Check sheet for the modelled part. Datum: model origin and axes. Units: mm. A direction names the side the tool comes from. Coordinates: 2 decimals unless noted, no trailing zeros. Write each loop counter-clockwise with the first axis right and the second up, starting at its lowest first coordinate (ties: lowest second). Pieces come first, ordered by that corner, then holes. Notation, with made-up numbers: M 43,28 L 84,28 A9 cw 84,44 Z; hole C 42.5,80 d7. An arc over 180 degrees is marked long. Answer as CSV lines item,"result". Start each with the question number.
Q1. Sectioned sample at D-D, the plane x = -24. Count the separate pieces of the cut face and the enclosed holes in it, then the cut area to 3 significant figures.
Q2. Sectioned sample at A-A, the plane y = -24. Record the cut outline in (x, z) (3 decimals), then the cut area to 3 significant figures.
Q3. Depth check by flat-ended pin: pin 1 Ø2 at (x, y) = (-29, -7.5) entering from +Z; pin 2 Ø1 at (x, z) = (-21.5, -27) entering from -Y; pin 3 Ø1.5 at (x, y) = (9.5, -14.5) entering from -Z. Enter the tip coordinate at first touch or a pass-through.
Q4. Mould release check, pull along Z, two halves, no side actions. Record for faces 4 (the flat face through (0, -15, 31.5)), 5 (the flat face through (-29, -7, 53.501)), 6 (the flat face through (20, -15, 10)), 7 (the flat face through (0.2, -26.25, 33.6)): pulls with the +Z half, pulls with the -Z half, needs draft (parallel to the pull), parting line crosses it, or undercut.
Q5. Sectioned sample at C-C, the plane y = -15.5. Record the cut outline in (x, z) (3 decimals).
Q6. Access from +Z, -Z, +X, -X, +Y, -Y to the whole of each face (thin tool, end or side, straight path). Record for faces 1 (the flat face through (29, -7, 53.501)), 2 (the flat face through (-23, -22, -13.501)), 3 (the cylindrical face through (0.06, -28.59, -23.75)).
Q7. Thickness scan on line 1 along X through (y, z) = (-23, 20) (3 decimals); line 2 along X through (y, z) = (-9.5, 37.5); line 3 along Z through (x, y) = (-22.5, -22). Record the ranges inside material, lowest first. Write a range as from..to.
Q8. Sectioned sample at B-B, the plane z = 20. Record the cut outline in (x, y) (3 decimals), then the cut area to 3 significant figures.
from build123d import *

# Parameters (mm, degrees)
SKETCH2_R           = 2.5
BOSS_EXTRUDE1_DEPTH = 3
BOSS_EXTRUDE2_DEPTH = 20
SKETCH4_R           = 2
BOSS_EXTRUDE3_DEPTH = 20
SKETCH6_R           = 4
BOSS_EXTRUDE5_DEPTH = 14
SKETCH7_W           = 28.258698574
SKETCH7_H           = 15
CUT_EXTRUDE1_DEPTH  = 9.25
FILLET1_R           = 30
SKETCH13_W          = 40
SKETCH13_H          = 40
BOSS_EXTRUDE8_DEPTH = 34
SKETCH14_R          = 2.875
CUT_EXTRUDE4_DEPTH  = 65.233633019
BOSS_EXTRUDE9_DEPTH = 20


with BuildPart() as part:
    # Sketch2 → Boss-Extrude1 (new body)
    with BuildSketch(Plane(origin=(0, 0, 0), x_dir=(1, 0, 0), z_dir=(0, 1, 0))):
        Polygon((-28, -11.5), (-20, -11.5), (-20, 10), (20, 10), (20, -11.5), (28, -11.5), (28, 11.5), (-28, 11.5), align=None)
        with Locations(Location((-24, 5, 0), (0, 0, 270))):
            Circle(SKETCH2_R, mode=Mode.SUBTRACT)
        with Locations(Location((-24, -5, 0), (0, 0, 90))):
            Circle(SKETCH2_R, mode=Mode.SUBTRACT)
        with Locations(Location((24, -5, 0), (0, 0, 270))):
            Circle(SKETCH2_R, mode=Mode.SUBTRACT)
        with Locations(Location((24, 5, 0), (0, 0, 90))):
            Circle(SKETCH2_R, mode=Mode.SUBTRACT)
    boss_extrude1 = extrude(amount=BOSS_EXTRUDE1_DEPTH)

    # Sketch3 → Boss-Extrude2 (add)
    with BuildSketch(Plane(origin=(0, 3, 0), x_dir=(1, 0, 0), z_dir=(0, 1, 0))):
        Polygon((-32.277683008, 10.5), (-32.277683008, -11.5), (-28, -11.5), (-28, 11.5), (28, 11.5), (28, -11.5), (32.493544997, -11.5), (32.493544997, 10.5), (32.493544997, 13.500761643), (-32.277683008, 13.500761643), align=None)
    boss_extrude2 = extrude(amount=-BOSS_EXTRUDE2_DEPTH)

    # Sketch4 → Boss-Extrude3 (add)
    with BuildSketch(Plane(origin=(0, 3, 0), x_dir=(1, 0, 0), z_dir=(0, 1, 0))):
        with BuildLine():
            Line((-3.795424266, 22.307494871), (-16.411972775, 11.5))
            Line((-16.411972775, 11.5), (16.493090482, 11.5))
            Line((16.493090482, 11.5), (4.035447529, 22.286686452))
            ThreePointArc((4.035447529, 22.286686452), (0.123874312, 23.75074046), (-3.795424266, 22.307494871))
        make_face()
        with Locations(Location((0.107930995, 17.750761643, 0), (0, 0, 270))):
            Circle(SKETCH4_R, mode=Mode.SUBTRACT)
    boss_extrude3 = extrude(amount=-BOSS_EXTRUDE3_DEPTH)

    # Sketch6 → Boss-Extrude5 (add)
    with BuildSketch(Plane.XZ.offset(17)):
        with BuildLine():
            Line((28, 11.5), (28, -11.5))
            Line((28, -11.5), (-28, -11.5))
            Line((-28, -11.5), (-28, 11.5))
            Line((-28, 11.5), (-32.277683008, 11.5))
            Line((-32.277683008, 11.5), (-32.277683008, -13.500761643))
            Line((-32.277683008, -13.500761643), (-14.076306034, -13.500761643))
            Line((-14.076306034, -13.500761643), (-3.795424266, -22.307494871))
            ThreePointArc((-3.795424266, -22.307494871), (0.123874312, -23.75074046), (4.035447529, -22.286686452))
            Line((4.035447529, -22.286686452), (14.18239254, -13.500761643))
            Line((14.18239254, -13.500761643), (32.493544997, -13.500761643))
            Line((32.493544997, -13.500761643), (32.493544997, 11.5))
            Line((32.493544997, 11.5), (28, 11.5))
        make_face()
        with Locations(Location((0.107930995, -17.750761643, 0), (0, 0, 270))):
            Circle(SKETCH6_R, mode=Mode.SUBTRACT)
    boss_extrude5 = extrude(amount=BOSS_EXTRUDE5_DEPTH)

    # Sketch7 → Cut-Extrude1 (cut)
    with BuildSketch(Plane(origin=(0, -17, 0), x_dir=(-1, 0, 0), z_dir=(0, -1, 0))):
        with Locations((-0.053043253, 19)):
            Rectangle(SKETCH7_W, SKETCH7_H)
    cut_extrude1 = extrude(amount=CUT_EXTRUDE1_DEPTH, mode=Mode.SUBTRACT)

    # Mirror1: Boss-Extrude1, Boss-Extrude2, Boss-Extrude3, Boss-Extrude5, Cut-Extrude1 across plane
    add(boss_extrude1.mirror(Plane.XY.offset(10)))
    add(boss_extrude2.mirror(Plane.XY.offset(10)))
    add(boss_extrude3.mirror(Plane.XY.offset(10)))
    add(boss_extrude5.mirror(Plane.XY.offset(10)))
    add(cut_extrude1.mirror(Plane.XY.offset(10)), mode=Mode.SUBTRACT)

    # Fillet1
    fillet1_edges = [part.edges().sort_by_distance(p)[0] for p in [
        (14.18239254, -28.625, -13.500761643),
        (-14.076306034, -7, -13.500761643),
        (14.18239254, -28.625, 33.500761643),
        (-14.076306034, -7, 33.500761643),
        (14.18239254, -7, 33.500761643),
        (-14.076306034, -28.625, 33.500761643),
        (-14.076306034, -28.625, -13.500761643),
        (14.18239254, -7, -13.500761643),
    ]]
    fillet(fillet1_edges, radius=FILLET1_R)

    # Sketch13 → Boss-Extrude8 (add)
    with BuildSketch(Plane(origin=(0, 3, 0), x_dir=(1, 0, 0), z_dir=(0, 1, 0))):
        with Locations((0, -10)):
            Rectangle(SKETCH13_W, SKETCH13_H)
    extrude(amount=-BOSS_EXTRUDE8_DEPTH)

    # Sketch14 → Cut-Extrude4 (cut, through all)
    with BuildSketch(Plane(origin=(0, 3, 0), x_dir=(1, 0, 0), z_dir=(0, 1, 0))):
        with Locations(Location((10, 0, 0), (0, 0, 270))):
            Circle(SKETCH14_R)
        with Locations(Location((10, -20, 0), (0, 0, 270))):
            Circle(SKETCH14_R)
    extrude(amount=-CUT_EXTRUDE4_DEPTH, mode=Mode.SUBTRACT)

    # Sketch15 → Boss-Extrude9 (add)
    with BuildSketch(Plane(origin=(0, 3, 0), x_dir=(1, 0, 0), z_dir=(0, 1, 0))):
        with BuildLine():
            ThreePointArc((25.365605991, -53.500761643), (21.872666456, -54.130629658), (18.8197451, -55.940886962))
            Line((18.8197451, -55.940886962), (17.127169311, -57.406435814))
            ThreePointArc((17.127169311, -57.406435814), (0.177018704, -63.750669852), (-16.806608467, -57.496605631))
            Line((-16.806608467, -57.496605631), (-18.663222883, -55.906206263))
            ThreePointArc((-18.663222883, -55.906206263), (-21.700786279, -54.121381232), (-25.168814984, -53.500761643))
            Line((-25.168814984, -53.500761643), (-32.277683008, -53.500761643))
            Line((-32.277683008, -53.500761643), (-32.277683008, -33.500761643))
            Line((-32.277683008, -33.500761643), (-25.168814984, -33.500761643))
            ThreePointArc((-25.168814984, -33.500761643), (-14.764728868, -35.362620409), (-5.652038682, -40.717095502))
            Line((-5.652038682, -40.717095502), (-3.795424266, -42.307494871))
            ThreePointArc((-3.795424266, -42.307494871), (0.123874312, -43.75074046), (4.035447529, -42.286686452))
            Line((4.035447529, -42.286686452), (5.728023318, -40.821137599))
            ThreePointArc((5.728023318, -40.821137599), (14.886787387, -35.39036569), (25.365605991, -33.500761643))
            Line((25.365605991, -33.500761643), (32.493544997, -33.500761643))
            Line((32.493544997, -33.500761643), (32.493544997, -53.500761643))
            Line((32.493544997, -53.500761643), (25.365605991, -53.500761643))
        make_face()
        with BuildLine():
            ThreePointArc((18.8197451, 35.940886962), (21.872666456, 34.130629658), (25.365605991, 33.500761643))
            Line((25.365605991, 33.500761643), (32.493544997, 33.500761643))
            Line((32.493544997, 33.500761643), (32.493544997, 13.500761643))
            Line((32.493544997, 13.500761643), (25.365605991, 13.500761643))
            ThreePointArc((25.365605991, 13.500761643), (14.886787387, 15.39036569), (5.728023318, 20.821137599))
            Line((5.728023318, 20.821137599), (4.035447529, 22.286686452))
            ThreePointArc((4.035447529, 22.286686452), (0.123874312, 23.75074046), (-3.795424266, 22.307494871))
            Line((-3.795424266, 22.307494871), (-5.652038682, 20.717095502))
            ThreePointArc((-5.652038682, 20.717095502), (-14.764728868, 15.362620409), (-25.168814984, 13.500761643))
            Line((-25.168814984, 13.500761643), (-32.277683008, 13.500761643))
            Line((-32.277683008, 13.500761643), (-32.277683008, 33.500761643))
            Line((-32.277683008, 33.500761643), (-25.168814984, 33.500761643))
            ThreePointArc((-25.168814984, 33.500761643), (-21.700786279, 34.121381232), (-18.663222883, 35.906206263))
            Line((-18.663222883, 35.906206263), (-16.806608467, 37.496605631))
            ThreePointArc((-16.806608467, 37.496605631), (0.177018704, 43.750669852), (17.127169311, 37.406435814))
            Line((17.127169311, 37.406435814), (18.8197451, 35.940886962))
        make_face()
    extrude(amount=-BOSS_EXTRUDE9_DEPTH)


solid = part.part
Output:
1,separate pieces,"5"
1,enclosed holes,"0"
1,area,"1,010 mm^2"
2,outline,"M -32.278,-13.501 L -14.076,-13.501 L -14.076,-11.5 L -28,-11.5 L -28,31.5 L -14.076,31.5 L -14.076,33.501 L -32.278,33.501 Z; M -20,-10 L 20,-10 L 20,30 L -20,30 Z; M 14.182,-13.501 L 32.494,-13.501 L 32.494,33.501 L 14.182,33.501 L 14.182,31.5 L 28,31.5 L 28,-11.5 L 14.182,-11.5 Z; hole C 10,0 d5.75; hole C 10,20 d5.75"
2,area,"2,070 mm^2"
3,pin 1,"stops at z = 53.5"
3,pin 2,"stops at y = -17"
3,pin 3,"stops at z = -42.27"
4,face 4,"undercut"
4,face 5,"pulls with the +Z half"
4,face 6,"undercut"
4,face 7,"needs draft"
5,outline,"M -32.278,-33.501 L -25.169,-33.501 A10 cw -18.663,-35.906 L -16.807,-37.497 A26 ccw 17.127,-37.406 L 18.82,-35.941 A10 cw 25.366,-33.501 L 32.494,-33.501 L 32.494,53.501 L 25.366,53.501 A10 cw 18.82,55.941 L 17.127,57.406 A26 ccw -16.807,57.497 L -18.663,55.906 A10 cw -25.169,53.501 L -32.278,53.501 Z; M -20,-10 L 20,-10 L 20,30 L -20,30 Z; hole M -28,-11.5 L 28,-11.5 L 28,31.5 L -28,31.5 Z; hole C 0.108,-17.751 d4; hole C 0.108,37.751 d4; hole C 10,0 d5.75; hole C 10,20 d5.75"
6,face 1,"+Z, +X, +Y, -Y"
6,face 2,"-Z, -X"
6,face 3,"-Z, -Y"
7,line 1,"x = -32.278..-28, -20..7.125, 12.875..20, 28..32.494"
7,line 2,"x = -32.28..-1.88, 2.09..32.49"
7,line 3,"z = -13.5..-11.5, 31.5..33.5"
8,outline,"M -32.278,-31 L -28,-31 L -28,0 L -20,0 L -20,-31 L 7.125,-31 L 7.125,3 L -32.278,3 Z; M 12.875,-31 L 20,-31 L 20,0 L 28,0 L 28,-31 L 32.494,-31 L 32.494,3 L 12.875,3 Z"
8,area,"1,510 mm^2"
